```python
from build123d import *

# Parameters (mm, degrees)
SKETCH1_R               = 30
BOSS_EXTRUDE1_DEPTH     = 10
SKETCH2_R               = 23.08
BOSS_EXTRUDE2_DEPTH     = 13.486192569
BOSS_EXTRUDE3_DEPTH     = 4
FILLET1_R               = 2
SKETCH5_R               = 1.5
CUT_EXTRUDE1_DEPTH      = 4
MIRROR2_COPY_1_SKETCH_R = 1.5
MIRROR2_COPY_1_DEPTH    = 4
FILLET1_OF_MIRROR2_R    = 2
SKETCH8_R               = 15
BOSS_EXTRUDE4_DEPTH     = 5
SKETCH13_R              = 2.5
BOSS_EXTRUDE6_DEPTH     = 10


with BuildPart() as part:
    # Sketch1 → Boss-Extrude1 (new body)
    with BuildSketch(Plane.XY):
        Circle(SKETCH1_R)
    extrude(amount=BOSS_EXTRUDE1_DEPTH)

    # Sketch2 → Boss-Extrude2 (add)
    with BuildSketch(Plane.XY.offset(10)):
        Circle(SKETCH2_R)
    extrude(amount=BOSS_EXTRUDE2_DEPTH)

    # Sketch4 → Boss-Extrude3 (add)
    with BuildSketch(Plane(origin=(0, 13, 0), x_dir=(1, 0, 0), z_dir=(0, 1, 0))):
        Polygon((28, -23.486192569), (-28, -23.486192569), (-36.579697763, -30.685413797), (-36.579697763, -35.685413797), (-23.08, -47.013005211), (23.08, -47.013005211), (36.579697763, -35.685413797), (36.579697763, -30.685413797), align=None)
    boss_extrude3 = extrude(amount=-BOSS_EXTRUDE3_DEPTH)

    # Fillet1
    fillet1_edges = [part.edges().sort_by_distance(p)[0] for p in [
        (-36.579697763, 11, 30.685413797),
        (-28, 11, 23.486192569),
        (28, 11, 23.486192569),
        (36.579697763, 11, 30.685413797),
        (36.579697763, 11, 35.685413797),
        (23.08, 11, 47.013005211),
        (-23.08, 11, 47.013005211),
        (-36.579697763, 11, 35.685413797),
    ]]
    fillet(fillet1_edges, radius=FILLET1_R)

    # Sketch5 → Cut-Extrude1 (cut)
    with BuildSketch(Plane(origin=(0, 13, 0), x_dir=(1, 0, 0), z_dir=(0, 1, 0))):
        with Locations(Location((-33.579697763, -33.185413797, 0), (0, 0, 270))):
            Circle(SKETCH5_R)
    cut_extrude1 = extrude(amount=-CUT_EXTRUDE1_DEPTH, mode=Mode.SUBTRACT)

    # Mirror1: Cut-Extrude1 across plane
    add(cut_extrude1.mirror(Plane(origin=(0, 0, 0), x_dir=(0, 0, 1), z_dir=(1, 0, 0))), mode=Mode.SUBTRACT)

    # Mirror2: Boss-Extrude3, Cut-Extrude1 across plane
    add(boss_extrude3.mirror(Plane.ZX))
    add(cut_extrude1.mirror(Plane.ZX), mode=Mode.SUBTRACT)

    # Mirror2 copy 1 sketch → Mirror2 copy 1 (cut)
    with BuildSketch(Plane(origin=(0, -13, 0), x_dir=(-1, 0, 0), z_dir=(0, -1, 0))):
        with Locations(Location((-33.579697763, -33.185413797, 0), (0, 0, 270))):
            Circle(MIRROR2_COPY_1_SKETCH_R)
    extrude(amount=-MIRROR2_COPY_1_DEPTH, mode=Mode.SUBTRACT)

    # Fillet1 of Mirror2
    fillet1_of_mirror2_edges = [part.edges().sort_by_distance(p)[0] for p in [
        (-36.579697763, -11, 30.685413797),
        (-28, -11, 23.486192569),
        (28, -11, 23.486192569),
        (36.579697763, -11, 30.685413797),
        (36.579697763, -11, 35.685413797),
        (23.08, -11, 47.013005211),
        (-23.08, -11, 47.013005211),
        (-36.579697763, -11, 35.685413797),
    ]]
    fillet(fillet1_of_mirror2_edges, radius=FILLET1_OF_MIRROR2_R)

    # Sketch8 → Boss-Extrude4 (add)
    with BuildSketch(Plane(origin=(0, 0, 0), x_dir=(-1, 0, 0), z_dir=(0, 0, -1))):
        with Locations(Location((0, 0, 0), (0, 0, 180))):
            Circle(SKETCH8_R)
    extrude(amount=BOSS_EXTRUDE4_DEPTH)

    # Sketch13 → Boss-Extrude6 (add)
    with BuildSketch(Plane(origin=(0, 0, -5), x_dir=(-1, 0, 0), z_dir=(0, 0, -1))):
        Circle(SKETCH13_R)
    extrude(amount=BOSS_EXTRUDE6_DEPTH)


solid = part.part
```
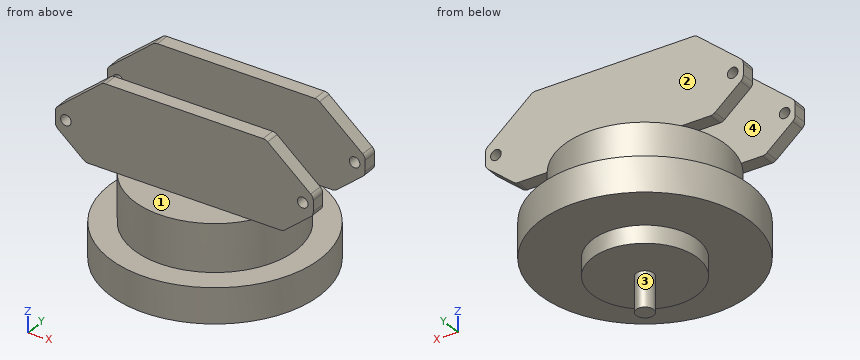
Can you work these out from the model? Positions are in its coordinate system, mm. Face numbers are marked on the shaded views. A direction names the side the tool comes from. Coordinates: 2 decimals unless noted, no trailing zeros. Loops run counter-clockwise (first coordinate to the right, second up) from the corner with the lowest first, then second, coordinate; pieces in that order, holes last. Notation, with made-up numbers: (89.5, 33.5) - (127.5, 33.5) arc R19 ccw to (127.5, 65.5) - close; hole circle Ø8 at (13.25, 55). An arc over 180 degrees is marked (long way). Use a Markdown table: item, result.
Item 1: For the marked faces 1, 2, 3 and 4, which set-ups out of +Z, -Z, +X, -X, +Y, -Y let a thin tool reach every point of the face, with its end or its side?
Numbers:
| item | result |
|---|---|
| face 1 | +Z, +X, -X, -Y |
| face 2 | +Z, +X, -X, +Y |
| face 3 | -Z |
| face 4 | +Z, +X, -X |
Item 2: I want a section at A-A on x = -26. Please give me the cut outline in (y, z), and give its area (3 significant figures).
Numbers:
| item | result |
|---|---|
| outline | (-14.97, 0) - (14.97, 0) - (14.97, 10) - (-14.97, 10) - close; (-13, 23.49) - (-9, 23.49) - (-9, 44.56) - (-13, 44.56) - close; (9, 23.49) - (13, 23.49) - (13, 44.56) - (9, 44.56) - close |
| area | 468 mm2 |
Item 3: I want a section at B-B on y = -11. Give the number of separate pieces and of enclosed holes in the cut face, and give its area (3 significant figures).
Numbers:
| item | result |
|---|---|
| separate pieces | 1 |
| enclosed holes | 2 |
| area | 2,700 mm2 |
Item 4: I want a section at C-C on z = 20. Please give me the cut outline in (x, y).
Numbers:
| item | result |
|---|---|
| outline | circle Ø46.16 at (0, 0) |
Item 5: Will these pins go through, and if not, where does the flat tip stop? pin 1 (2 mm diameter, centred on x = 2, y = -23.5, fed in from +Z); pin 2 (7 mm diameter, centred on x = 13.5, z = 37.5, fed in from -Y); pin 3 (3 mm diameter, centred on x = -25, y = -10, fed in from -Z); pin 4 (1.8 mm diameter, centred on x = -33.58, z = 33.19, fed in from -Y).
Numbers:
| item | result |
|---|---|
| pin 1 | stops at z = 23.49 |
| pin 2 | stops at y = -13 |
| pin 3 | stops at z = 0 |
| pin 4 | passes through |
Item 6: I want a section at D-D on x = 0. Please give me the cut outline in (y, z).
Numbers:
| item | result |
|---|---|
| outline | (-30, 0) - (-15, 0) - (-15, -5) - (-2.5, -5) - (-2.5, -15) - (2.5, -15) - (2.5, -5) - (15, -5) - (15, 0) - (30, 0) - (30, 10) - (23.08, 10) - (23.08, 23.49) - (13, 23.49) - (13, 47.01) - (9, 47.01) - (9, 23.49) - (-9, 23.49) - (-9, 47.01) - (-13, 47.01) - (-13, 23.49) - (-23.08, 23.49) - (-23.08, 10) - (-30, 10) - close |
Item 7: If I drill on probe 1 along Z at (x, y) = (-21, -10); probe 2 along Y at (x, z) = (20, 33); probe 3 along Z at (x, y) = (18.5, 23.5), over which ranges is the centre line in solid material (lowest first)? Write a range as from..to.
Numbers:
| item | result |
|---|---|
| probe 1 | z = 0..10, 23.49..47.01 |
| probe 2 | y = -13..-9, 9..13 |
| probe 3 | z = 0..10 |
